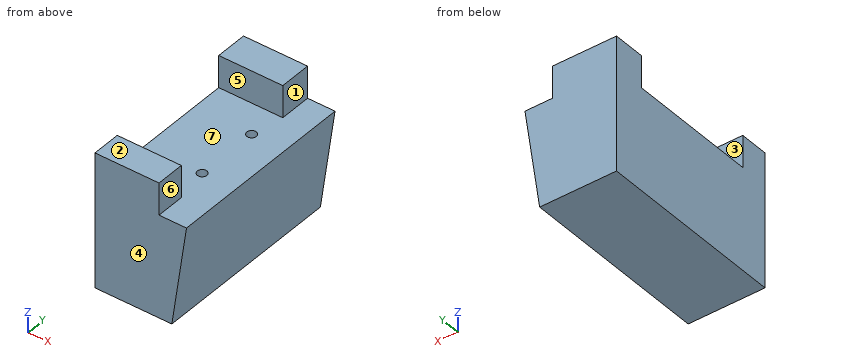
from build123d import *

# Parameters (mm, degrees)
F1_DEPTH = 30
F2_R     = 0.75
F3_DEPTH = 10
F4_W     = 10
F4_H     = 5
F4_H_2   = 4.5
F5_DEPTH = 5


# Not quite as in the source:
# - a feature names something its author has since deleted; it is built from what else it names


with BuildPart() as f1:
    # F0 (on Front) → F1 (new body)
    with BuildSketch(Plane.XZ):
        Polygon((0, 16), (0, 0), (12, 0), (14.29, 16), align=None)
    extrude(amount=F1_DEPTH)

    # F2 (on face) → F3 (cut)
    with BuildSketch(Plane.XY.offset(16)):
        with Locations((9, -10)):
            Circle(F2_R)
        with Locations((9, -20)):
            Circle(F2_R)
    extrude(amount=-F3_DEPTH, mode=Mode.SUBTRACT)

    # F4 (on face) → F5 (join)
    with BuildSketch(Plane.XY.offset(16)):
        with Locations((5, -2.5)):
            Rectangle(F4_W, F4_H)
        with Locations((5, -27.75)):
            Rectangle(F4_W, F4_H_2)
    extrude(amount=F5_DEPTH)


solid = f1.part
The listing builds one solid part. Answer for the finished solid, in the listing's coordinates (mm). Face numbers are marked on the shaded views. A direction names the side the tool comes from. Coordinates: 2 decimals unless noted, no trailing zeros. Write each loop counter-clockwise with the first axis right and the second up, starting at its lowest first coordinate (ties: lowest second). Pieces come first, ordered by that corner, then holes. Notation, with made-up numbers: (54.5, -23.75) -> (80.5, -23.75) arc R24 cw to (80.5, 8.25) -> close; hole circle Ø11 at (-3.5, 50). An arc over 180 degrees is marked (long way). One line per question, with ' | ' between items.
1. Section D-D (z = 7.75) is taken. Determine the outline of the cut face in (x, y), and give its area (3 significant figures).
Verdict:
outline: (0, -30) -> (13.11, -30) -> (13.11, 0) -> (0, 0) -> close; hole circle Ø1.5 at (9, -20); hole circle Ø1.5 at (9, -10) | area: 390 mm^2
2. Which of the six approach directions +Z, -Z, +X, -X, +Y, -Y give full straight-line access (tool end or side, diameter ignored) to the marked faces 1, 2 and 3?
Verdict:
face 1: +Z, +X, +Y, -Y | face 2: +Z, +X, -X, +Y, -Y | face 3: +Z, +X, -X
3. Given pin 1 Ø2 at (y, z) = (-8.5, 4) entering from -X; pin 2 Ø2 at (y, z) = (-28, 18.5) entering from +X; pin 3 Ø2 at (x, y) = (9, -10) entering from +Z, each flat-ended and moving along its own axis, determine where each tip first touches the part or whether it passes through.
Verdict:
pin 1: stops at x = 0 | pin 2: stops at x = 10 | pin 3: stops at z = 16
4. Section C-C (y = -20) is taken. Determine the outline of the cut face in (x, z), and give its area (3 significant figures).
Verdict:
outline: (0, 0) -> (12, 0) -> (14.29, 16) -> (9.75, 16) -> (9.75, 6) -> (8.25, 6) -> (8.25, 16) -> (0, 16) -> close | area: 195 mm^2
5. Section A-A (z = 19.25) is taken. Determine the outline of the cut face in (x, y).
Verdict:
outline: (0, -30) -> (10, -30) -> (10, -25.5) -> (0, -25.5) -> close; (0, -5) -> (10, -5) -> (10, 0) -> (0, 0) -> close
6. For a pull along Y with two mould halves and no side action, classify the marked faces 4, 5, 6 and 7 as released by +Y, released by -Y, zero draft, split by the parting line, or undercut.
Verdict:
face 4: released by -Y | face 5: undercut | face 6: zero draft | face 7: undercut
7. Section B-B (x = 9) is taken. Determine the outline of the cut face in (y, z).
Verdict:
outline: (-30, 0) -> (0, 0) -> (0, 21) -> (-5, 21) -> (-5, 16) -> (-9.25, 16) -> (-9.25, 6) -> (-10.75, 6) -> (-10.75, 16) -> (-19.25, 16) -> (-19.25, 6) -> (-20.75, 6) -> (-20.75, 16) -> (-25.5, 16) -> (-25.5, 21) -> (-30, 21) -> close
8. Straight lines are drawn through the part: line 1 (Y direction, x = 9, z = 14); line 2 (Y direction, x = 5, z = 18.25); line 3 (Z direction, x = 3.25, y = -21.25). For each, find the intervals that lie inside material, in ascending order.
Verdict:
line 1: y = -30 to -20.75, -19.25 to -10.75, -9.25 to 0 | line 2: y = -30 to -25.5, -5 to 0 | line 3: z = 0 to 16
